from build123d import *

# Parameters (mm, degrees)
F0_W     = 65
F0_H     = 55
F0_W_2   = 61
F0_H_2   = 51
F1_DEPTH = 2.5
F2_DEPTH = 10
F3_R     = 2
F4_R     = 4
F7_R     = 1


with BuildPart() as f1:
    # F0 (on Top) → F1 (new body)
    with BuildSketch(Plane.XY):
        Rectangle(F0_W, F0_H)
        Rectangle(F0_W_2, F0_H_2, mode=Mode.SUBTRACT)
        Rectangle(F0_W_2, F0_H_2)
        with BuildLine():
            ThreePointArc((-26, 18), (-24.75, 19.25), (-23.5, 18))
            Line((-23.5, 18), (-23.5, -18))
            ThreePointArc((-23.5, -18), (-24.75, -19.25), (-26, -18))
            Line((-26, -18), (-26, 18))
        make_face(mode=Mode.SUBTRACT)
        with BuildLine():
            Line((-19.5, -18), (-19.5, 18))
            ThreePointArc((-19.5, 18), (-18.25, 19.25), (-17, 18))
            Line((-17, 18), (-17, -18))
            ThreePointArc((-17, -18), (-18.25, -19.25), (-19.5, -18))
        make_face(mode=Mode.SUBTRACT)
        with BuildLine():
            Line((-13, -18), (-13, 18))
            ThreePointArc((-13, 18), (-11.75, 19.25), (-10.5, 18))
            Line((-10.5, 18), (-10.5, -18))
            ThreePointArc((-10.5, -18), (-11.75, -19.25), (-13, -18))
        make_face(mode=Mode.SUBTRACT)
        with BuildLine():
            Line((-6.5, -18), (-6.5, 18))
            ThreePointArc((-6.5, 18), (-5.25, 19.25), (-4, 18))
            Line((-4, 18), (-4, -18))
            ThreePointArc((-4, -18), (-5.25, -19.25), (-6.5, -18))
        make_face(mode=Mode.SUBTRACT)
        with BuildLine():
            Line((4, -18), (4, 18))
            ThreePointArc((4, 18), (5.25, 19.25), (6.5, 18))
            Line((6.5, 18), (6.5, -18))
            ThreePointArc((6.5, -18), (5.25, -19.25), (4, -18))
        make_face(mode=Mode.SUBTRACT)
        with BuildLine():
            Line((10.5, -18), (10.5, 18))
            ThreePointArc((10.5, 18), (11.75, 19.25), (13, 18))
            Line((13, 18), (13, -18))
            ThreePointArc((13, -18), (11.75, -19.25), (10.5, -18))
        make_face(mode=Mode.SUBTRACT)
        with BuildLine():
            ThreePointArc((17, 18), (18.25, 19.25), (19.5, 18))
            Line((19.5, 18), (19.5, -18))
            ThreePointArc((19.5, -18), (18.25, -19.25), (17, -18))
            Line((17, -18), (17, 18))
        make_face(mode=Mode.SUBTRACT)
        with BuildLine():
            Line((23.5, -18), (23.5, 18))
            ThreePointArc((23.5, 18), (24.75, 19.25), (26, 18))
            Line((26, 18), (26, -18))
            ThreePointArc((26, -18), (24.75, -19.25), (23.5, -18))
        make_face(mode=Mode.SUBTRACT)
    extrude(amount=F1_DEPTH)

    # F0 (on Top) → F2 (join)
    with BuildSketch(Plane.XY):
        Rectangle(F0_W, F0_H)
        Rectangle(F0_W_2, F0_H_2, mode=Mode.SUBTRACT)
    extrude(amount=F2_DEPTH)

    # F3
    f3_edges = [f1.edges().sort_by_distance(p)[0] for p in [
        (-30.5, 25.5, 6.25),
        (30.5, 25.5, 6.25),
        (-30.5, -25.5, 6.25),
        (30.5, -25.5, 6.25),
    ]]
    fillet(f3_edges, radius=F3_R)

    # F4
    f4_edges = [f1.edges().sort_by_distance(p)[0] for p in [
        (-32.5, 27.5, 5),
        (32.5, 27.5, 5),
        (-32.5, -27.5, 5),
        (32.5, -27.5, 5),
    ]]
    fillet(f4_edges, radius=F4_R)

    # F6: sweep along a path in F6_path
    with BuildLine(Plane(origin=(-30.5, 23.5, 10), x_dir=(0, 1, 0), z_dir=(0, 0, 1))) as f6_path:
        Line((0, 0), (-47, 0))
        ThreePointArc((-47, 0), (-48.4142135624, -0.5857864376), (-49, -2))
        Line((-49, -2), (-49, -59))
        ThreePointArc((-49, -59), (-48.4142135624, -60.4142135624), (-47, -61))
        Line((-47, -61), (0, -61))
        ThreePointArc((0, -61), (1.4142135624, -60.4142135624), (2, -59))
        Line((2, -59), (2, -2))
        ThreePointArc((2, -2), (1.4142135624, -0.5857864376), (0, 0))
    # F5 (on Front) → F6 (sweep)
    with BuildSketch(Plane.XZ):
        with BuildLine():
            Line((-30.5, 10), (-30.5, 6.2521283853))
            Line((-30.5, 6.2521283853), (-29.8801235899, 7.9552248249))
            ThreePointArc((-29.8801235899, 7.9552248249), (-29.85, 8.1260641927), (-29.8801235899, 8.2969035604))
            Line((-29.8801235899, 8.2969035604), (-30.5, 10))
        make_face()
    sweep(path=f6_path.line)

    # F7
    f7_edges = [f1.edges().sort_by_distance(p)[0] for p in [
        (0, 27.5, 10),
    ]]
    fillet(f7_edges, radius=F7_R)


solid = f1.part
Model file for the job. Use its own axes, mm. A direction names the side the tool comes from. Give positions to 0.01 mm unless a question says otherwise; leave off trailing zeros. Order: outer loops, then holes, each group sorted by start corner. A loop starts at its lowest first (then second) coordinate and runs counter-clockwise, first axis right, second up. Notation, with made-up numbers: M 37.5,3.25 L 96.5,3.25 A11 cw 96.5,9.25 Z; hole C 14.5,30 d7. An arc over 180 degrees is marked long. Put each result on its own line as item: value. Start each with the question number.
(1) Tool access for faces 4 (the face through (0.399, -25.186, 9.137)), 5 (the face through (0, 26, 10)), 6 (the face through (-17, 0, 1)), 7 (the face through (-29.705, -24.679, 7.116)): list every direction of +Z, -Z, +X, -X, +Y, -Y with a clear straight run to the whole face (end or side of a thin tool).
(2) Drill centre lines: L1, parallel to Y at x = -2, z = 8.25; L2, parallel to Y at x = -11.5, z = 3; L3, parallel to X at y = 20, z = 6. Where is each one in solid material? Low to high. Write a range as [from, to].
(3) Pull direction Y, two halves, no side cores. Call faces 1 (the face through (-31.359, -26.297, 4.563)), 2 (the face through (29.685, -24.711, 9.16)), 3 (the face through (-31.359, 26.297, 4.437)): released by +Y, released by -Y, zero draft, split by the parting line, or undercut.
(4) Band-saw the part on D-D on x = -16. Give the cut face in (y, z), then the cut area to 3 significant figures.
(5) Band-saw the part on A-A on z = 4.5. Give the cut face in (x, y).
(6) Band-saw the part on B-B on x = -24.75. Give the cut face in (y, z).
(7) Band-saw the part on C-C on y = 1. Count the separate pieces of the cut face and the enclosed holes in it, then the cut area to 3 significant figures.
Results below:
1. face 4: +Z
1. face 5: +Z, +X, -X, +Y, -Y
1. face 6: +Z, -Z
1. face 7: none
2. L1: y = [-27.5, -24.87], [24.87, 27.5]
2. L2: y = [-27.5, -25.5], [25.5, 27.5]
2. L3: x = [-32.5, -30.5], [30.5, 32.5]
3. face 1: released by -Y
3. face 2: undercut
3. face 3: released by +Y
4. outline: M -27.5,0 L 27.5,0 L 27.5,9 A1 ccw 26.5,10 L 25.5,10 L 24.88,8.3 A0.5 ccw 24.88,7.96 L 25.5,6.25 L 25.5,2.5 L -25.5,2.5 L -25.5,6.25 L -24.88,7.96 A0.5 ccw -24.88,8.3 L -25.5,10 L -26.5,10 A1 ccw -27.5,9 Z
4. area: 170 mm2
5. outline: M -32.5,-23.5 A4 ccw -28.5,-27.5 L 28.5,-27.5 A4 ccw 32.5,-23.5 L 32.5,23.5 A4 ccw 28.5,27.5 L -28.5,27.5 A4 ccw -32.5,23.5 Z; hole M -30.5,-23.5 A2 ccw -28.5,-25.5 L 28.5,-25.5 A2 ccw 30.5,-23.5 L 30.5,23.5 A2 ccw 28.5,25.5 L -28.5,25.5 A2 ccw -30.5,23.5 Z
6. outline: M -27.5,0 L -19.25,0 L -19.25,2.5 L -25.5,2.5 L -25.5,6.25 L -24.88,7.96 A0.5 ccw -24.88,8.3 L -25.5,10 L -26.5,10 A1 ccw -27.5,9 Z; M 19.25,0 L 27.5,0 L 27.5,9 A1 ccw 26.5,10 L 25.5,10 L 24.88,8.3 A0.5 ccw 24.88,7.96 L 25.5,6.25 L 25.5,2.5 L 19.25,2.5 Z
7. separate pieces: 9
7. enclosed holes: 0
7. area: 145 mm2
